Here's how the part is built. I have some questions about the finished solid (model axes, mm). A direction names the side the tool comes from. Coordinates: 2 decimals unless noted, no trailing zeros. Write each loop counter-clockwise with the first axis right and the second up, starting at its lowest first coordinate (ties: lowest second). Pieces come first, ordered by that corner, then holes. Notation, with made-up numbers: (86.25, 76) -> (107.25, 76) arc R29 cw to (107.25, 97) -> close; hole circle Ø1 at (41, 73.25). An arc over 180 degrees is marked (long way). Use a Markdown table: item, result. Add a question column.
Item 1: On a 3-axis mill with a long thin cutter (end or side, diameter ignored), from which of +Z, -Z, +X, -X, +Y, -Y can I reach the whole of each face in a straight line? I mean faces 1 (the flat face through (76.311, 4.93, -60.107)), 2 (the flat face through (-49.689, 4.93, -60.107)), 3 (the flat face through (79, 5, 21.366)), 4 (the flat face through (82.7, 4.9, 14.9)), 5 (the flat face through (17, 1, -51.134)). Say none if no direction works.
Item 2: Imagine slicing it at B-B, the plane x = -23.5. Write out the boundary of the cut face in (y, z), and give its area (3 significant figures).
Item 3: Imagine slicing it at C-C, the plane z = -28.5. Write out the boundary of the cut face in (x, y), and give its area (3 significant figures).
Item 4: If I drill on line 1 along Z through (x, y) = (77.5, 5); line 2 along X through (y, z) = (0.25, -54); line 3 along Y through (x, z) = (20.5, -24.5), over which ranges is the centre line in solid material (lowest first)? Write a range as from..to.
Item 5: Will these pins go through, and if not, where does the flat tip stop? pin 1 Ø2.5 at (x, y) = (58.5, 2) entering from +Z; pin 2 Ø3 at (x, z) = (55.5, -56) entering from +Y; pin 3 Ø2.5 at (x, y) = (61, 1.5) entering from -Z.
Item 6: If we mould it in two halves opening along Z, with no side actions, what happens to faces 6 (the flat face through (16, 0, -21)), 7 (the flat face through (-27, 1, -51.134)), 8 (the flat face through (-49.72, 4.93, 19.78)), 9 (the flat face through (5.468, 1.479, -56.064))? For each: pulls with the +Z half, pulls with the -Z half, needs draft (parallel to the pull), parting line crosses it, or undercut.
Item 7: Imagine slicing it at A-A, the plane y = 5. Count the separate pieces of the cut face and the enclosed holes in it, and give its area (3 significant figures).
```python
from build123d import *

# Parameters (mm, degrees)
SKETCH3_W           = 140
SKETCH3_H           = 89
BOSS_EXTRUDE1_DEPTH = 3
SKETCH2_W           = 111
SKETCH2_H           = 10
BOSS_EXTRUDE3_DEPTH = 3
BOSS_EXTRUDE4_DEPTH = 10
SKETCH4_R           = 1.9
CUT_EXTRUDE1_DEPTH  = 141


with BuildPart() as part:
    # Sketch3 → Boss-Extrude1 (new body)
    with BuildSketch(Plane(origin=(0, 0, 0), x_dir=(1, 0, 0), z_dir=(0, 1, 0))):
        with Locations((16.502784142, 20.134430227)):
            Rectangle(SKETCH3_W, SKETCH3_H)
    extrude(amount=-BOSS_EXTRUDE1_DEPTH)

    # Sketch2 → Boss-Extrude3 (add)
    with BuildSketch(Plane(origin=(0, 0, 0), x_dir=(1, 0, 0), z_dir=(0, 1, 0))):
        Polygon((-38.901339061, 51.134430227), (-37.138069254, 61.134430227), (-16.919207001, 61.134430227), (-15.155937194, 51.134430227), align=None)
        Polygon((26.580792999, 61.134430227), (28.344062806, 51.134430227), (4.598660939, 51.134430227), (6.361930746, 61.134430227), align=None)
        Polygon((70.080792999, 61.134430227), (71.844062806, 51.134430227), (48.098660939, 51.134430227), (49.861930746, 61.134430227), align=None)
        with Locations((16.502784142, -15.865569773)):
            Rectangle(SKETCH2_W, SKETCH2_H)
    extrude(amount=BOSS_EXTRUDE3_DEPTH)

    # Sketch2_4 → Boss-Extrude4 (add)
    with BuildSketch(Plane(origin=(0, 0, 0), x_dir=(1, 0, 0), z_dir=(0, 1, 0))):
        Polygon((-44.187814781, -13.365569773), (-48.806616934, -13.365569773), (-51.116018011, -17.365569773), (-48.806616934, -21.365569773), (-44.187814781, -21.365569773), (-41.878413704, -17.365569773), align=None)
        Polygon((-48.806616934, 53.634430227), (-44.187814781, 53.634430227), (-41.878413704, 57.634430227), (-44.187814781, 61.634430227), (-48.806616934, 61.634430227), (-51.116018011, 57.634430227), align=None)
        Polygon((74.883981989, 57.634430227), (77.193383066, 53.634430227), (81.812185219, 53.634430227), (84.121586296, 57.634430227), (81.812185219, 61.634430227), (77.193383066, 61.634430227), align=None)
        Polygon((81.812185219, -21.365569773), (84.121586296, -17.365569773), (81.812185219, -13.365569773), (77.193383066, -13.365569773), (74.883981989, -17.365569773), (77.193383066, -21.365569773), align=None)
    extrude(amount=BOSS_EXTRUDE4_DEPTH)

    # Sketch4 → Cut-Extrude1 (cut, through all)
    with BuildSketch(Plane.ZY.offset(53.497215858)):
        with Locations((-57.634430227, 5)):
            Circle(SKETCH4_R)
        with Locations((17.365569773, 5)):
            Circle(SKETCH4_R)
    extrude(amount=-CUT_EXTRUDE1_DEPTH, mode=Mode.SUBTRACT)


solid = part.part
```
Ans:
| question | item | result |
|---|---|---|
| 1 | face 1 | -Z, +Y |
| 1 | face 2 | -Z, -X, +Y |
| 1 | face 3 | +Z, +X, -X, +Y |
| 1 | face 4 | +X, +Y |
| 1 | face 5 | +X, -X, +Y |
| 2 | outline | (-3, -64.63) -> (0, -64.63) -> (0, -61.13) -> (3, -61.13) -> (3, -51.13) -> (0, -51.13) -> (0, 10.87) -> (3, 10.87) -> (3, 20.87) -> (0, 20.87) -> (0, 24.37) -> (-3, 24.37) -> close |
| 2 | area | 327 mm^2 |
| 3 | outline | (-53.5, -3) -> (86.5, -3) -> (86.5, 0) -> (-53.5, 0) -> close |
| 3 | area | 420 mm^2 |
| 4 | line 1 | z = -61.63..-59.53, -55.73..-53.63, 13.37..15.47, 19.27..21.37 |
| 4 | line 2 | x = -49.02..-43.98, -38.4..-15.66, 5.1..27.84, 48.6..71.34, 76.98..82.02 |
| 4 | line 3 | y = -3..0 |
| 5 | pin 1 | stops at z = 20.87 |
| 5 | pin 2 | stops at y = 3 |
| 5 | pin 3 | stops at z = -61.13 |
| 6 | face 6 | undercut |
| 6 | face 7 | undercut |
| 6 | face 8 | pulls with the +Z half |
| 6 | face 9 | pulls with the -Z half |
| 7 | separate pieces | 8 |
| 7 | enclosed holes | 0 |
| 7 | area | 98.0 mm^2 |
